Read the model definition and answer for the solid it produces. Units are mm, in the model's axes. Round coordinates to 2 decimals unless told otherwise and drop trailing zeros. Loops run counter-clockwise (first coordinate to the right, second up) from the corner with the lowest first, then second, coordinate; pieces in that order, holes last. Notation, with made-up numbers: (16.5, 44.5) - (62.5, 44.5) arc R24 ccw to (62.5, 76.5) - close; hole circle Ø9 at (60.5, -2.75). An arc over 180 degrees is marked (long way). Use one line per item in the form item = value. Start each with the question number.
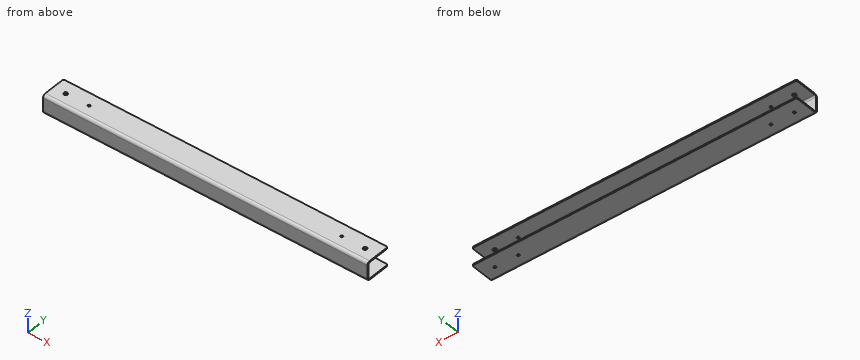
```python
from build123d import *

# Parameters (mm, degrees)
SKETCH1_W                            = 660.4
SKETCH1_H                            = 38.1
BASE_FLANGE1_DEPTH                   = 2.65684
EDGE_FLANGE1_STRIP_W                 = 16.97736
EDGE_FLANGE1_STRIP_H                 = 2.65684
EDGE_FLANGE1_STRIP_CUT_DEPTH         = 660.4
EDGE_FLANGE1_STRIP_2_W               = 16.97736
EDGE_FLANGE1_STRIP_2_H               = 2.65684
EDGE_FLANGE1_STRIP_CUT_2_DEPTH       = 660.4
EDGE_FLANGE1_DEPTH                   = 660.4
EDGE_FLANGE1_BEND_DEPTH              = 660.4
F_10_0_1935_DIAMETER_HOLE2_D         = 4.9149
F_10_0_1935_DIAMETER_HOLE2_DEPTH     = 2.65684
FILLET1_R                            = 3.175
F_10_0_1935_DIAMETER_HOLE3_D         = 4.9149
F_19_64_0_29688_DIAMETER_HOLE1_D     = 7.540752
F_19_64_0_29688_DIAMETER_HOLE1_DEPTH = 2.65684


# Sheet-metal steps are written as plain solids
with BuildPart() as part:
    # Sketch1 → Base-Flange1 (new body)
    with BuildSketch(Plane(origin=(0, 0, 0), x_dir=(1, 0, 0), z_dir=(0, 1, 0))):
        with Locations((375.92, 15.875)):
            Rectangle(SKETCH1_W, SKETCH1_H)
    extrude(amount=-BASE_FLANGE1_DEPTH)

    # Edge-Flange1 strip (across the edge) → Edge-Flange1 strip cut (cut)
    with BuildSketch(Plane(origin=(45.72, 0, 3.175), x_dir=(0, 0, -1), z_dir=(1, 0, 0))):
        with Locations((-2.65684, -1.32842)):
            Rectangle(EDGE_FLANGE1_STRIP_W, EDGE_FLANGE1_STRIP_H)
    extrude(amount=EDGE_FLANGE1_STRIP_CUT_DEPTH, mode=Mode.SUBTRACT)

    # Edge-Flange1 strip 2 (across the edge) → Edge-Flange1 strip cut 2 (cut)
    with BuildSketch(Plane(origin=(706.12, 0, -34.925), x_dir=(0, 0, 1), z_dir=(-1, 0, 0))):
        with Locations((-2.65684, -1.32842)):
            Rectangle(EDGE_FLANGE1_STRIP_2_W, EDGE_FLANGE1_STRIP_2_H)
    extrude(amount=EDGE_FLANGE1_STRIP_CUT_2_DEPTH, mode=Mode.SUBTRACT)

    # Edge-Flange1 section (across the edge) → Edge-Flange1 (add)
    with BuildSketch(Plane(origin=(45.72, 0, 3.175), x_dir=(0, 0, -1), z_dir=(1, 0, 0))):
        with BuildLine():
            Line((0, 3.175), (0, 48.14316))
            Line((0, 48.14316), (2.65684, 48.14316))
            Line((2.65684, 48.14316), (2.65684, 3.175))
            ThreePointArc((2.65684, 3.175), (3.58677597, 0.92993597), (5.83184, 0))
            Line((5.83184, 0), (5.83184, -2.65684))
            ThreePointArc((5.83184, -2.65684), (1.708106389, -0.948733611), (0, 3.175))
        make_face()
    extrude(amount=EDGE_FLANGE1_DEPTH)

    # Edge-Flange1 section 2 (across the edge) → Edge-Flange1 bend (add)
    with BuildSketch(Plane(origin=(706.12, 0, -34.925), x_dir=(0, 0, 1), z_dir=(-1, 0, 0))):
        with BuildLine():
            Line((0, 3.175), (0, 48.14316))
            Line((0, 48.14316), (2.65684, 48.14316))
            Line((2.65684, 48.14316), (2.65684, 3.175))
            ThreePointArc((2.65684, 3.175), (3.58677597, 0.92993597), (5.83184, 0))
            Line((5.83184, 0), (5.83184, -2.65684))
            ThreePointArc((5.83184, -2.65684), (1.708106389, -0.948733611), (0, 3.175))
        make_face()
    extrude(amount=EDGE_FLANGE1_BEND_DEPTH)

    # #10 (0.1935) Diameter Hole2
    with Locations(Plane(origin=(0, 0, -34.925), x_dir=(-1, 0, 0), z_dir=(0, 0, -1))):
        with Locations((-680.72, 22.74316), (-633.095, 22.74316), (-118.745, 22.74316), (-71.12, 22.74316)):
            Hole(F_10_0_1935_DIAMETER_HOLE2_D / 2, depth=F_10_0_1935_DIAMETER_HOLE2_DEPTH)

    # Fillet1
    fillet1_edges = [part.edges().sort_by_distance(p)[0] for p in [
        (45.72, 48.14316, 1.84658),
        (706.12, 48.14316, 1.84658),
        (706.12, 48.14316, -33.59658),
        (45.72, 48.14316, -33.59658),
    ]]
    fillet(fillet1_edges, radius=FILLET1_R)

    # #10 (0.1935) Diameter Hole3 (through all)
    with Locations(Plane.XY.offset(3.175)):
        with Locations((633.095, 22.74316), (118.745, 22.74316)):
            Hole(F_10_0_1935_DIAMETER_HOLE3_D / 2)

    # 19/64 (0.29688) Diameter Hole1
    with Locations(Plane.XY.offset(3.175)):
        with Locations((71.12, 22.74316), (680.72, 22.74316)):
            Hole(F_19_64_0_29688_DIAMETER_HOLE1_D / 2, depth=F_19_64_0_29688_DIAMETER_HOLE1_DEPTH)


solid = part.part
```
1) Straight lines are drawn through the part: line 1 (Z direction, x = 594, y = 45) (3 decimals); line 2 (Y direction, x = 125.5, z = -27); line 3 (Y direction, x = 544, z = -2). For each, find the intervals that lie inside material, in ascending order. Write a range as from..to.
2) A cutting plane is placed at C-C on z = -9.5. Write down the section's boundary in (x, y).
3) A flat-ended cylindrical pin translates along its axis: pin 1 (21 mm diameter, centred on x = 268.5, z = -18.5, fed in from +Y). Find the tip coordinate at first contact, or state that the pin passes through.
4) A cutting plane is placed at B-B on x = 613. Write down the section's boundary in (y, z) (3 decimals).
5) A cutting plane is placed at A-A on y = 9.5. Write down the section's boundary in (x, z) (3 decimals).
Checks:
q1.line_1 = -34.925..-32.268, 0.518..3.175
q1.line_2 = -2.66..0
q1.line_3 = -2.62..0.07
q2.outline = (45.72, -2.66) - (706.12, -2.66) - (706.12, 0) - (45.72, 0) - close
q3.pin_1 = 0
q4.outline = (-2.657, -29.093) arc R5.832 ccw to (3.175, -34.925) - (48.143, -34.925) - (48.143, -32.268) - (3.175, -32.268) arc R3.175 cw to (0, -29.093) - (0, -2.657) arc R3.175 cw to (3.175, 0.518) - (48.143, 0.518) - (48.143, 3.175) - (3.175, 3.175) arc R5.832 ccw to (-2.657, -2.657) - close
q5.outline = (45.72, -34.925) - (706.12, -34.925) - (706.12, -32.268) - (45.72, -32.268) - close; (45.72, 0.518) - (706.12, 0.518) - (706.12, 3.175) - (45.72, 3.175) - close
